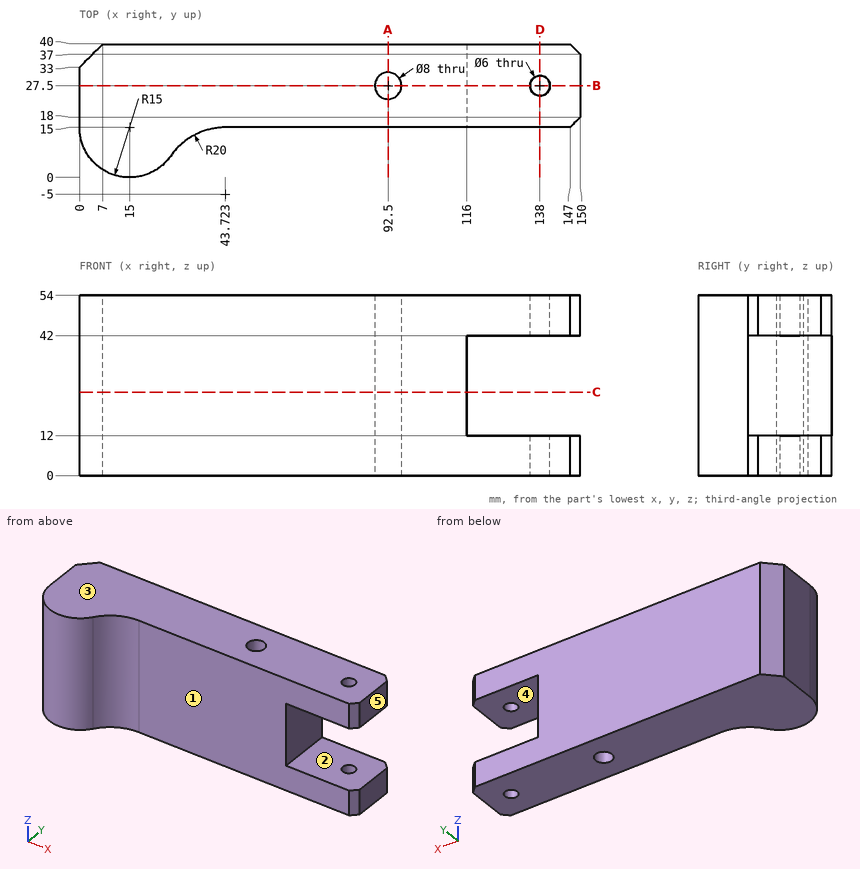
For this review, use the dimensioned drawing (mm, ordinates from the lowest corner) and the shaded views. A direction names the side the tool comes from. Coordinates: 2 decimals unless noted, no trailing zeros. Order: outer loops, then holes, each group sorted by start corner. A loop starts at its lowest first (then second) coordinate and runs counter-clockwise, first axis right, second up. Notation, with made-up numbers: (70, 71.25) - (129, 71.25) arc R19 cw to (129, 102.25) - close; hole circle Ø5 at (63, -25.75). An arc over 180 degrees is marked (long way). Answer in a Markdown table with one row per item.
(1) The part is to be moulded in two halves that separate along Z. For the marked faces 1, 2 and 3, say which applies: released by +Z, released by -Z, zero draft, split by the parting line, or undercut.
Checked values:
| item | result |
|---|---|
| face 1 | zero draft |
| face 2 | undercut |
| face 3 | released by +Z |
(2) Consider section A-A on x = 92.5. State the section outline as (y, z) points.
Checked values:
| item | result |
|---|---|
| outline | (15, 0) - (23.5, 0) - (23.5, 54) - (15, 54) - close; (31.5, 0) - (40, 0) - (40, 54) - (31.5, 54) - close |
(3) Clearance check with flat-ended pins moving along their axes: pin 1 (2 mm diameter, centred on x = 26.5, z = 35, fed in from -Y); pin 2 (12.5 mm diameter, centred on y = 29.5, z = 29, fed in from +X). State where each tip first meets the part, or that it passes through.
Checked values:
| item | result |
|---|---|
| pin 1 | y = 4.29 |
| pin 2 | x = 116 |
(4) Consider section C-C on z = 25. State the section outline as (x, y) points.
Checked values:
| item | result |
|---|---|
| outline | (0, 15) arc R15 ccw to (27.31, 6.43) arc R20 cw to (43.72, 15) - (116, 15) - (116, 40) - (7, 40) - (0, 33) - close; hole circle Ø8 at (92.5, 27.5) |
(5) Consider section D-D on x = 138. State the section outline as (y, z) points, plus the area to 3 significant figures.
Checked values:
| item | result |
|---|---|
| outline | (15, 0) - (24.5, 0) - (24.5, 12) - (15, 12) - close; (15, 42) - (24.5, 42) - (24.5, 54) - (15, 54) - close; (30.5, 0) - (40, 0) - (40, 12) - (30.5, 12) - close; (30.5, 42) - (40, 42) - (40, 54) - (30.5, 54) - close |
| area | 456 mm^2 |
(6) Consider section B-B on y = 27.5. State the section outline as (x, z) points.
Checked values:
| item | result |
|---|---|
| outline | (0, 0) - (88.5, 0) - (88.5, 54) - (0, 54) - close; (96.5, 0) - (135, 0) - (135, 12) - (116, 12) - (116, 42) - (135, 42) - (135, 54) - (96.5, 54) - close; (141, 0) - (150, 0) - (150, 12) - (141, 12) - close; (141, 42) - (150, 42) - (150, 54) - (141, 54) - close |
(7) For the marked faces 4 and 5, list the 3-axis set-ups (+Z, -Z, +X, -X, +Y, -Y) from which the entire face can be reached by the end or side of a thin tool; tool diameter is ignored.
Checked values:
| item | result |
|---|---|
| face 4 | +X, +Y, -Y |
| face 5 | +Z, -Z, +X, +Y, -Y |
(8) Wall thickness on line 1 along Y through (x, z) = (138, 6); line 2 along X through (y, z) = (27.5, 48); line 3 along Y through (x, z) = (92, 29): over which ranges is each line inside the solid? List them lowest first. Write a range as from..to.
Checked values:
| item | result |
|---|---|
| line 1 | 15..24.5, 30.5..40 |
| line 2 | 0..88.5, 96.5..135, 141..150 |
| line 3 | 15..23.53, 31.47..40 |
